```python
from build123d import *

# Parameters (mm, degrees)
F1_DEPTH = 21.43125
F2_R     = 9.525
F3_DEPTH = 50.8
F4_R     = 1.5875
F6_DEPTH = 42.8635
F7_DEPTH = 55.1070625421


with BuildPart() as f1:
    # F0 (on Right) → F1 (new body, symmetric)
    with BuildSketch(Plane.YZ):
        Polygon((-152.4, 69.85), (-152.4, 0), (152.4, 0), (152.4, 19.05), align=None)
    extrude(amount=F1_DEPTH, both=True)

    # F2 (on face) → F3 (cut)
    with BuildSketch(Plane.XZ.offset(152.4)):
        with Locations((0, 34.925)):
            Circle(F2_R)
    extrude(amount=-F3_DEPTH, mode=Mode.SUBTRACT)

    # F4 (on face) → F6 (intersect, through all)
    with BuildSketch(Plane.YZ.offset(21.43125)):
        with BuildLine():
            Line((-149.7065071007, 50.8408099003), (-152.4, 50.7999993861))
            Line((-152.4, 50.7999993861), (-152.4, 0))
            Line((-152.4, 0), (57.15, 0))
            add(Edge.make_bspline(
                [(57.15, 27.6693087071), (62.9540532827, 23.1574121863), (64.8345353288, 15.2838414165), (60.2900164004, 5.1415623251), (57.15, 0)],
                knots=[0, 0, 0, 0, 0.4816979855, 1, 1, 1, 1], degree=3))
            add(Edge.make_bspline(
                [(-27.3415464908, 40.8684164286), (-8.4446382918, 39.1311924639), (24.8142205738, 35.0208202174), (47.8670857847, 31.8072736263), (57.15, 27.6693087071)],
                knots=[0, 0, 0, 0, 0.5631768545, 1, 1, 1, 1], degree=3))
            add(Edge.make_bspline(
                [(-27.3415464908, 40.8684164286), (-35.3624819778, 44.1492309528), (-56.5713824039, 52.8243373258), (-104.2014900273, 51.7497373627), (-133.8184987721, 51.0815373923)],
                knots=[0, 0, 0, 0, 0.3781872386, 1, 1, 1, 1], degree=3))
            Line((-133.8184987721, 51.0815373923), (-152.4, 55.1060624421))
            Line((-152.4, 55.1060624421), (-149.7065071007, 50.8408099003))
        make_face()
        with Locations((-126.3143569231, 9.525)):
            Circle(F4_R, mode=Mode.SUBTRACT)
        with Locations((29.0634203702, 9.525)):
            Circle(F4_R, mode=Mode.SUBTRACT)
    extrude(amount=-F6_DEPTH, mode=Mode.INTERSECT)

    # F5 (on face) → F7 (intersect, through all)
    with BuildSketch(Plane(origin=(0, 0, 0), x_dir=(1, 0, 0), z_dir=(0, 0, -1))):
        with BuildLine():
            add(Edge.make_bspline(
                [(-21.43125, 141.3332819939), (-21.105100692, 143.7924098417), (-19.7181081761, 148.2729204744), (-18.7462978065, 151.51001513), (-15.875, 152.4)],
                knots=[0, 0, 0, 0, 0.5247215937, 1, 1, 1, 1], degree=3))
            Line((-21.43125, 141.3332819939), (-21.43125, 39.6870598197))
            add(Edge.make_bspline(
                [(-21.43125, 39.6870598197), (-19.8348436954, 15.699516797), (-18.7155051196, -26.3628345266), (-16.2676267963, -47.1015389649), (-10.981831047, -64.1384903262), (0, -64.5855814219)],
                knots=[0, 0, 0, 0, 0.4656404532, 0.7315566193, 1, 1, 1, 1], degree=3))
            add(Edge.make_bspline(
                [(21.43125, 39.6870598197), (19.8348436954, 15.699516797), (18.7155051196, -26.3628345266), (16.2676267963, -47.1015389649), (10.981831047, -64.1384903262), (0, -64.5855814219)],
                knots=[0, 0, 0, 0, 0.4656404532, 0.7315566193, 1, 1, 1, 1], degree=3))
            Line((21.43125, 39.6870598197), (21.43125, 141.3332819939))
            add(Edge.make_bspline(
                [(21.43125, 141.3332819939), (21.105100692, 143.7924098417), (19.7181081761, 148.2729204744), (18.7462978065, 151.51001513), (15.875, 152.4)],
                knots=[0, 0, 0, 0, 0.5247215937, 1, 1, 1, 1], degree=3))
            Line((15.875, 152.4), (-15.875, 152.4))
        make_face()
    extrude(amount=-F7_DEPTH, mode=Mode.INTERSECT)


solid = f1.part
```
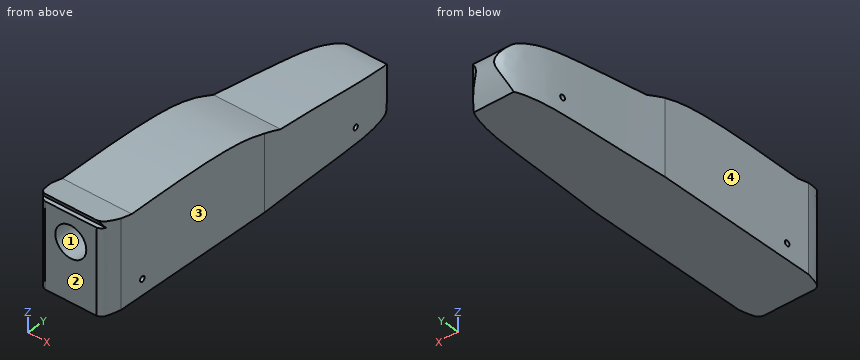
Geometry: final body of the model. Coordinates: model frame, mm. Face numbers are marked on the shaded views. Round coordinates to 2 decimals unless told otherwise and drop trailing zeros. Use one line per item in the form item = value.
(1) Section A-A on x = 0. Count the separate pieces of the cut face and the enclosed holes in it, and give its area (3 significant figures).
Results list:
separate_pieces = 1
enclosed_holes = 2
area = 8,430 mm^2
(2) First-contact query: pin 1 Ø15 at (x, z) = (0, 34.925) entering from +Y; pin 2 Ø12 at (y, z) = (-18.5, 28) entering from +X; pin 3 Ø12 at (x, y) = (-10, 8.5) entering from +Z. Flat tips, straight axial feed; report the tip coordinate or a pass-through.
Results list:
pin_1 = 57.46
pin_2 = 20.54
pin_3 = 37.7
(3) Ray query, probe 1 along Y at (x, z) = (6.5, 9.5); probe 2 along X at (y, z) = (4.5, 18); probe 3 along Z at (x, y) = (-6.5, -137.5). Return the intervals inside material, ascending. Write a range as [from, to].
Results list:
probe_1 = [-152.4, -127.9], [-124.73, 27.48], [30.65, 61.85]
probe_2 = [-19.22, 19.22]
probe_3 = [0, 27.96], [41.89, 51.88]
(4) Draft query along X for the marked faces 1, 2, 3 and 4. Return one class per face: pulls with the +X half, pulls with the -X half, needs draft (parallel to the pull), parting line crosses it, or undercut.
Results list:
face_1 = undercut
face_2 = needs draft
face_3 = pulls with the +X half
face_4 = pulls with the -X half
